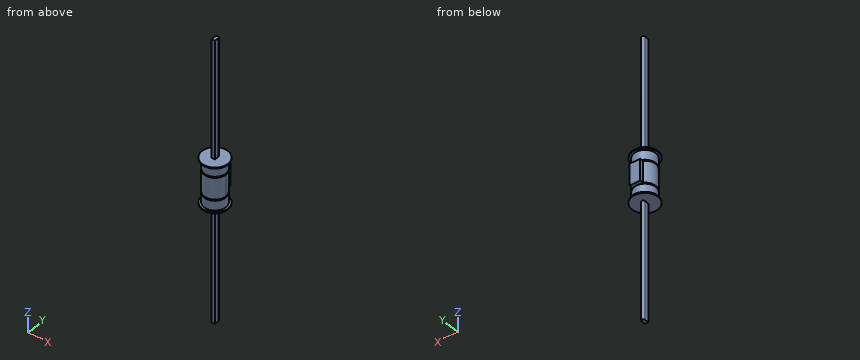
from build123d import *

# Parameters (mm, degrees)
BOSS_EXTRUDE4_DEPTH = 55
SKETCH4_R           = 5
BOSS_EXTRUDE5_DEPTH = 5
BOSS_EXTRUDE6_DEPTH = 10
SKETCH6_R           = 5
BOSS_EXTRUDE7_DEPTH = 5
BOSS_EXTRUDE8_DEPTH = 55
CUT_EXTRUDE2_START  = -0.5
SKETCH8_R           = 5
SKETCH8_R_2         = 4.5
CUT_EXTRUDE2_DEPTH  = 0.5
SKETCH9_R           = 6
BOSS_EXTRUDE9_DEPTH = 0.5


with BuildPart() as part:
    # Sketch1 → Boss-Extrude4 (new body)
    with BuildSketch(Plane.XY):
        with BuildLine():
            ThreePointArc((-0.75, 1), (0, 0.25), (0.75, 1))
            Line((0.75, 1), (-0.75, 1))
        make_face()
        with BuildLine():
            Line((-0.75, 1), (0.75, 1))
            ThreePointArc((0.75, 1), (0, 1.75), (-0.75, 1))
        make_face()
        with BuildLine():
            Line((-0.75, -1), (0.75, -1))
            Line((0.75, -1), (0.75, 1))
            ThreePointArc((0.75, 1), (0, 0.25), (-0.75, 1))
            Line((-0.75, 1), (-0.75, -1))
        make_face()
    extrude(amount=BOSS_EXTRUDE4_DEPTH)

    # Sketch4 → Boss-Extrude5 (add)
    with BuildSketch(Plane.XY.offset(55)):
        Circle(SKETCH4_R)
    extrude(amount=BOSS_EXTRUDE5_DEPTH)

    # Sketch5 → Boss-Extrude6 (add)
    with BuildSketch(Plane.XY.offset(60)):
        with BuildLine():
            Line((2.5, 4.330127019), (2.5, 4))
            Line((2.5, 4), (-2.5, 4))
            Line((-2.5, 4), (-2.5, 4.330127019))
            ThreePointArc((-2.5, 4.330127019), (-2.5, -4.330127019), (5, 0))
            ThreePointArc((5, 0), (4.330127019, 2.5), (2.5, 4.330127019))
        make_face()
        with BuildLine():
            Line((-2.5, 4), (2.5, 4))
            Line((2.5, 4), (2.5, 4.330127019))
            ThreePointArc((2.5, 4.330127019), (0, 5), (-2.5, 4.330127019))
            Line((-2.5, 4.330127019), (-2.5, 4))
        make_face()
        with BuildLine():
            ThreePointArc((-2.5, 4.330127019), (0, 5), (2.5, 4.330127019))
            Line((2.5, 4.330127019), (2.5, 6))
            Line((2.5, 6), (-2.5, 6))
            Line((-2.5, 6), (-2.5, 4.330127019))
        make_face()
    extrude(amount=BOSS_EXTRUDE6_DEPTH)

    # Sketch6 → Boss-Extrude7 (add)
    with BuildSketch(Plane.XY.offset(70)):
        Circle(SKETCH6_R)
    extrude(amount=BOSS_EXTRUDE7_DEPTH)

    # Sketch7 → Boss-Extrude8 (add)
    with BuildSketch(Plane.XY.offset(75)):
        with BuildLine():
            ThreePointArc((-0.75, 1), (0, 0.25), (0.75, 1))
            Line((0.75, 1), (-0.75, 1))
        make_face()
        with BuildLine():
            Line((-0.75, 1), (0.75, 1))
            ThreePointArc((0.75, 1), (0, 1.75), (-0.75, 1))
        make_face()
        with BuildLine():
            Line((-0.75, -1), (0.75, -1))
            Line((0.75, -1), (0.75, 1))
            ThreePointArc((0.75, 1), (0, 0.25), (-0.75, 1))
            Line((-0.75, 1), (-0.75, -1))
        make_face()
    extrude(amount=BOSS_EXTRUDE8_DEPTH)

    # Sketch8 → Cut-Extrude2 (cut)
    with BuildSketch(Plane.XY.offset(60).offset(CUT_EXTRUDE2_START)):
        Circle(SKETCH8_R)
        Circle(SKETCH8_R_2, mode=Mode.SUBTRACT)
    cut_extrude2 = extrude(amount=CUT_EXTRUDE2_DEPTH, mode=Mode.SUBTRACT)

    # Mirror3: Cut-Extrude2 across plane
    add(cut_extrude2.mirror(Plane.XY.offset(65)), mode=Mode.SUBTRACT)

    # Sketch9 → Boss-Extrude9 (add)
    with BuildSketch(Plane(origin=(0, 0, 55), x_dir=(-1, 0, 0), z_dir=(0, 0, -1))):
        Circle(SKETCH9_R)
    boss_extrude9 = extrude(amount=BOSS_EXTRUDE9_DEPTH)

    # Mirror4: Boss-Extrude9 across plane
    add(boss_extrude9.mirror(Plane.XY.offset(65)))


solid = part.part
Geometry check sheet. Reference: the model listing, model coordinates, mm. Round coordinates to 2 decimals unless told otherwise and drop trailing zeros. Loops run counter-clockwise (first coordinate to the right, second up) from the corner with the lowest first, then second, coordinate; pieces in that order, holes last. Notation, with made-up numbers: (43.5, 87.25) -> (81.5, 87.25) arc R23 cw to (81.5, 100.25) -> close; hole circle Ø5 at (40.25, -29.75). An arc over 180 degrees is marked (long way). Answer as a JSON object with one key per item and string values. Group by question number.
Item 1: Cross-section at A-A, the plane y = 3. Record the cut outline in (x, z).
Item 2: Cross-section at B-B, the plane z = 73.5. Record the cut outline in (x, y), plus the area to 3 significant figures.
Item 3: Depth check by flat-ended pin: pin 1 Ø0.6 at (y, z) = (0, 105) entering from -X; pin 2 Ø5 at (y, z) = (3.5, 66.5) entering from +X; pin 3 Ø6 at (y, z) = (1.5, 102) entering from +X; pin 4 Ø6 at (x, y) = (-2.5, 2.5) entering from +Z. Enter the tip coordinate at first touch or a pass-through.
Item 4: Thickness scan on line 1 along Z through (x, y) = (-0.25, -4.75); line 2 along Z through (x, y) = (-4.5, -3.5); line 3 along Z through (x, y) = (-3.5, 0.25). Record the ranges inside material, lowest first.
Determined:
{
 "1": {"outline": "(-5.2, 54.5) -> (5.2, 54.5) -> (5.2, 55) -> (4, 55) -> (4, 59.5) -> (3.35, 59.5) -> (3.35, 60) -> (4, 60) -> (4, 70) -> (3.35, 70) -> (3.35, 70.5) -> (4, 70.5) -> (4, 75) -> (5.2, 75) -> (5.2, 75.5) -> (-5.2, 75.5) -> (-5.2, 75) -> (-4, 75) -> (-4, 70.5) -> (-3.35, 70.5) -> (-3.35, 70) -> (-4, 70) -> (-4, 60) -> (-3.35, 60) -> (-3.35, 59.5) -> (-4, 59.5) -> (-4, 55) -> (-5.2, 55) -> close"},
 "2": {"outline": "circle Ø10 at (0, 0)", "area": "78.5 mm²"},
 "3": {"pin 1": "stops at x = -0.75", "pin 2": "stops at x = 4.9", "pin 3": "stops at x = 0.75", "pin 4": "stops at z = 130"},
 "4": {"line 1": "z = 54.5 to 59.5, 60 to 70, 70.5 to 75.5", "line 2": "z = 54.5 to 55, 75 to 75.5", "line 3": "z = 54.5 to 75.5"}
}
